Answer from the drawing. Dimensions are ordinates in mm from the lowest x, y and z of the part. Coordinates: 2 decimals unless noted, no trailing zeros. Write each loop counter-clockwise with the first axis right and the second up, starting at its lowest first coordinate (ties: lowest second). Pieces come first, ordered by that corner, then holes.
(1) Given pin 1 (10 mm diameter, centred on x = 59, y = 27.5, fed in from -Z), flat-ended and moving along its own axis, determine where the tip first touches the part or whether it passes through.
(2) Section A-A on x = 35 is taken. Write down the section's boundary in (y, z).
(3) Section C-C on z = 0.25 is taken. Write down the section's boundary in (x, y).
(4) Section D-D on x = 27 is taken. Write down the section's boundary in (y, z).
(5) Find the intervals of material crossed by probe 1 along X at (y, z) = (18, 0.35) (1 decimal); probe 2 along Y at (x, z) = (35, 0.8); probe 3 along X at (y, z) = (20.5, 0.35), in increasing order.
(6) Section B-B on y = 20 is taken. Write down the section's boundary in (x, z), then the cut area to 3 significant figures.
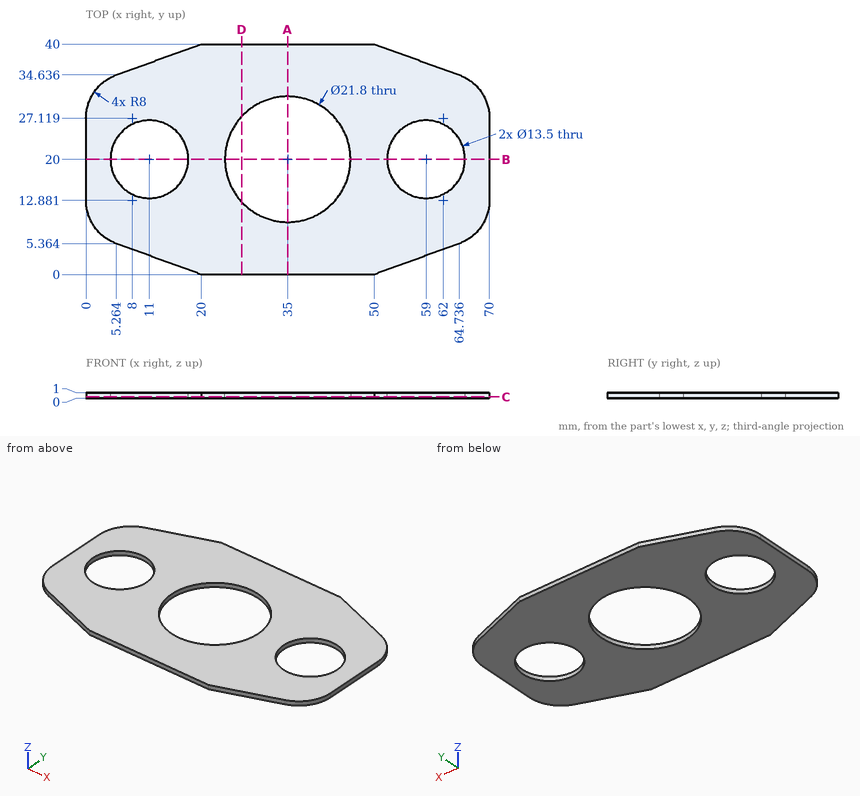
Response:
1. pin 1: stops at z = 0
2. outline: (0, 0) - (9.1, 0) - (9.1, 1) - (0, 1) - close; (30.9, 0) - (40, 0) - (40, 1) - (30.9, 1) - close
3. outline: (0, 12.88) arc R8 ccw to (5.26, 5.36) - (20, 0) - (50, 0) - (64.74, 5.36) arc R8 ccw to (70, 12.88) - (70, 27.12) arc R8 ccw to (64.74, 34.64) - (50, 40) - (20, 40) - (5.26, 34.64) arc R8 ccw to (0, 27.12) - close; hole circle Ø13.5 at (11, 20); hole circle Ø21.8 at (35, 20); hole circle Ø13.5 at (59, 20)
4. outline: (0, 0) - (12.6, 0) - (12.6, 1) - (0, 1) - close; (27.4, 0) - (40, 0) - (40, 1) - (27.4, 1) - close
5. probe 1: x = 0 to 4.6, 17.4 to 24.3, 45.7 to 52.6, 65.4 to 70
5. probe 2: y = 0 to 9.1, 30.9 to 40
5. probe 3: x = 0 to 4.27, 17.73 to 24.11, 45.89 to 52.27, 65.73 to 70
6. outline: (0, 0) - (4.25, 0) - (4.25, 1) - (0, 1) - close; (17.75, 0) - (24.1, 0) - (24.1, 1) - (17.75, 1) - close; (45.9, 0) - (52.25, 0) - (52.25, 1) - (45.9, 1) - close; (65.75, 0) - (70, 0) - (70, 1) - (65.75, 1) - close
6. area: 21.2 mm2
